The listing builds one solid part. Answer for the finished solid, in the listing's coordinates (mm). Coordinates: 2 decimals unless noted, no trailing zeros. Write each loop counter-clockwise with the first axis right and the second up, starting at its lowest first coordinate (ties: lowest second). Pieces come first, ordered by that corner, then holes. Notation, with made-up numbers: M 18.25,42.5 L 45.25,42.5 A16 ccw 45.25,50.5 Z; hole C 34.5,-6.75 d2. An arc over 180 degrees is marked long. Write item = value, one per line. Start each with the question number.
```python
from build123d import *

# Parameters (mm, degrees)
F1_DEPTH = 3


with BuildPart() as f1:
    # F0 (on Front) → F1 (new body)
    with BuildSketch(Plane.XZ):
        with BuildLine():
            ThreePointArc((-41.5685183068, 17.2115741473), (-31.7863073381, 15.2891766842), (-41.5685183068, 13.3667792212))
            Line((-41.5685183068, 13.3667792212), (-41.5685183068, 6.2897060804))
            add(Edge.make_bspline(
                [(-41.5685183068, 6.2897060804), (-40.5110451617, 4.3618677361), (-38.4157281513, 0.5419764273), (-34.1862913757, 0.1795269801), (-32.091384023, 0)],
                knots=[0, 0, 0, 0, 0.5046840835, 1, 1, 1, 1], degree=3))
            Line((-32.091384023, 0), (7.2702049994, 0))
            add(Edge.make_bspline(
                [(15.2129016184, 5.3413121865), (14.6447493994, 3.7606222596), (13.4476780972, 0.4301793154), (9.3978891034, 0.1481650631), (7.2702049994, 0)],
                knots=[0, 0, 0, 0, 0.4746185277, 1, 1, 1, 1], degree=3))
            Line((15.2129016184, 5.3413121865), (15.2129016184, 12.6273036262))
            ThreePointArc((15.2129016184, 12.6273036262), (5.4398618144, 14.5719828795), (15.2129016184, 16.5166621327))
            Line((15.2129016184, 16.5166621327), (15.2129016184, 23.8026535724))
            add(Edge.make_bspline(
                [(15.2129016184, 23.8026535724), (15.1610136829, 25.4929601247), (15.0013770651, 30.6932984806), (2.0501826306, 30.6246729843), (-6.691384023, 30.5783533685)],
                knots=[0, 0, 0, 0, 0.3250378027, 1, 1, 1, 1], degree=3))
            Line((-6.691384023, 30.5783533685), (-32.091384023, 30.5783533685))
            add(Edge.make_bspline(
                [(-41.5685183068, 24.288647288), (-40.9100897642, 25.9794911706), (-39.4843435822, 29.6408060352), (-34.6780612652, 30.2503206867), (-32.091384023, 30.5783533685)],
                knots=[0, 0, 0, 0, 0.4618132953, 1, 1, 1, 1], degree=3))
            Line((-41.5685183068, 24.288647288), (-41.5685183068, 17.2115741473))
        make_face()
    extrude(amount=F1_DEPTH)


solid = f1.part
```
1. For a pull along Z with two mould halves and no side action, classify faces 1 (the face through (5.444, -1.479, 14.377)), 2 (the face through (-13, -1, 0)), 3 (the face through (-31.79, -1.48, 15.48)), 4 (the face through (15.213, -1, 9)) as pulls with the +Z half, pulls with the -Z half, needs draft (parallel to the pull), parting line crosses it, or undercut.
2. Straight lines are drawn through the part: L1, parallel to X at y = -2.55, z = 18; L2, parallel to X at y = -1.7, z = 12; L3, parallel to Z at x = -4.5, y = -2.05. For each, find the intervals that lie inside material, in ascending order. Write a range as [from, to].
3. The part is cut by section A-A, the plane z = 19. Write down the section's boundary in (x, y), and give its area (3 significant figures).
Solution:
q1.face_1 = undercut
q1.face_2 = pulls with the -Z half
q1.face_3 = undercut
q1.face_4 = needs draft
q2.L1 = [-41.57, -41.16], [-32.57, 6.77], [14.27, 15.21]
q2.L2 = [-41.57, -40.74], [-32.99, 6.14], [14.9, 15.21]
q2.L3 = [0, 30.59]
q3.outline = M -41.57,-3 L -40.34,-3 L -40.34,0 L -41.57,0 Z; M -33.4,-3 L 8.03,-3 L 8.03,0 L -33.4,0 Z; M 13.01,-3 L 15.21,-3 L 15.21,0 L 13.01,0 Z
q3.area = 135 mm^2
